from build123d import *

# Parameters (mm, degrees)
STOCK_HORN_DRIVE_FLANGE_START              = 41
STOCK_HORN_DRIVE_FLANGE_PROFILE_R          = 13
STOCK_HORN_DRIVE_FLANGE_PROFILE_R_2        = 4.05
STOCK_HORN_DRIVE_FLANGE_DEPTH              = 3
D_COUPLING_RING_START                      = 44
D_COUPLING_RING_PROFILE_R                  = 7
D_COUPLING_RING_PROFILE_R_2                = 4.05
D_COUPLING_RING_DEPTH                      = 4
D_KEY_LAND_START                           = 44
D_KEY_LAND_PROFILE_W                       = 2.9
D_KEY_LAND_PROFILE_H                       = 4.8
D_KEY_LAND_DEPTH                           = 4
CAPTURED_HORN_KEY_BOSS_START               = 39.35
CAPTURED_HORN_KEY_BOSS_PROFILE_R           = 13
CAPTURED_HORN_KEY_BOSS_DEPTH               = 1.65
KEY_POCKET_HUB_START                       = 39.35
STOCK_HORN_POCKET_HUB_R                    = 3.55
KEY_POCKET_HUB_DEPTH                       = 1.65
KEY_POCKET_HORIZONTAL_START                = 39.35
STOCK_HORN_POCKET_HORIZONTAL_W             = 16.3
STOCK_HORN_POCKET_HORIZONTAL_H             = 4.2
KEY_POCKET_HORIZONTAL_DEPTH                = 1.65
KEY_POCKET_VERTICAL_START                  = 39.35
STOCK_HORN_POCKET_VERTICAL_W               = 4.2
STOCK_HORN_POCKET_VERTICAL_H               = 16.3
KEY_POCKET_VERTICAL_DEPTH                  = 1.65
KEY_POCKET_ROUNDED_TIPS_START              = 39.35
STOCK_HORN_POCKET_ROUNDED_TIPS_R           = 2.1
KEY_POCKET_ROUNDED_TIPS_DEPTH              = 1.65
UNMODIFIED_HORN_CAPTURE_M2_START           = -50
UNMODIFIED_HORN_CAPTURE_M2_PROFILE_R       = 1.15
UNMODIFIED_HORN_CAPTURE_M2_DEPTH           = 102.400389104
HUB_CLEARANCE_IN_KEY_BOSS_ONLY_START       = 39.35
HORN_CENTER_HUB_CLEARANCE_R                = 4
HUB_CLEARANCE_IN_KEY_BOSS_ONLY_DEPTH       = 1.65
YAW_POSITIVE_RETENTION_CROSSBOLT_START     = -10
YAW_POSITIVE_RETENTION_CROSSBOLT_PROFILE_R = 1.1
YAW_POSITIVE_RETENTION_CROSSBOLT_DEPTH     = 62.400389104
CROSSBOLT_FLAT_SEAT_CUT_12_START           = -12
CROSSBOLT_FLAT_SEAT_12_R                   = 2.75
CROSSBOLT_FLAT_SEAT_CUT_12_DEPTH           = 6
CROSSBOLT_FLAT_SEAT_CUT_6_START            = 6
CROSSBOLT_FLAT_SEAT_6_R                    = 2.75
CROSSBOLT_FLAT_SEAT_CUT_6_DEPTH            = 6


with BuildPart() as part:
    # Stock_horn_drive_flange_profile → Stock_horn_drive_flange (new body)
    with BuildSketch(Plane(origin=(0, 0, 0), x_dir=(1, 0, 0), z_dir=(0, 1, 0)).offset(STOCK_HORN_DRIVE_FLANGE_START)):
        with Locations(Location((0, 0, 0), (0, 0, 270))):
            Circle(STOCK_HORN_DRIVE_FLANGE_PROFILE_R)
        with Locations(Location((0, 0, 0), (0, 0, 270))):
            Circle(STOCK_HORN_DRIVE_FLANGE_PROFILE_R_2, mode=Mode.SUBTRACT)
    extrude(amount=STOCK_HORN_DRIVE_FLANGE_DEPTH)

    # D_coupling_ring_profile → D_coupling_ring (add)
    with BuildSketch(Plane(origin=(0, 0, 0), x_dir=(1, 0, 0), z_dir=(0, 1, 0)).offset(D_COUPLING_RING_START)):
        with Locations(Location((0, 0, 0), (0, 0, 270))):
            Circle(D_COUPLING_RING_PROFILE_R)
        with Locations(Location((0, 0, 0), (0, 0, 270))):
            Circle(D_COUPLING_RING_PROFILE_R_2, mode=Mode.SUBTRACT)
    extrude(amount=D_COUPLING_RING_DEPTH)

    # D_key_land_profile → D_key_land (add)
    with BuildSketch(Plane(origin=(0, 0, 0), x_dir=(1, 0, 0), z_dir=(0, 1, 0)).offset(D_KEY_LAND_START)):
        with Locations((4.55, 0)):
            Rectangle(D_KEY_LAND_PROFILE_W, D_KEY_LAND_PROFILE_H)
    extrude(amount=D_KEY_LAND_DEPTH)

    # Captured_horn_key_boss_profile → Captured_horn_key_boss (add)
    with BuildSketch(Plane(origin=(0, 0, 0), x_dir=(1, 0, 0), z_dir=(0, 1, 0)).offset(CAPTURED_HORN_KEY_BOSS_START)):
        with Locations(Location((0, 0, 0), (0, 0, 270))):
            Circle(CAPTURED_HORN_KEY_BOSS_PROFILE_R)
    extrude(amount=CAPTURED_HORN_KEY_BOSS_DEPTH)

    # Stock_horn_pocket_Hub → Key_pocket_Hub (cut)
    with BuildSketch(Plane(origin=(0, 0, 0), x_dir=(1, 0, 0), z_dir=(0, 1, 0)).offset(KEY_POCKET_HUB_START)):
        with Locations(Location((0, 0, 0), (0, 0, 270))):
            Circle(STOCK_HORN_POCKET_HUB_R)
    extrude(amount=KEY_POCKET_HUB_DEPTH, mode=Mode.SUBTRACT)

    # Stock_horn_pocket_Horizontal → Key_pocket_Horizontal (cut)
    with BuildSketch(Plane(origin=(0, 0, 0), x_dir=(1, 0, 0), z_dir=(0, 1, 0)).offset(KEY_POCKET_HORIZONTAL_START)):
        Rectangle(STOCK_HORN_POCKET_HORIZONTAL_W, STOCK_HORN_POCKET_HORIZONTAL_H)
    extrude(amount=KEY_POCKET_HORIZONTAL_DEPTH, mode=Mode.SUBTRACT)

    # Stock_horn_pocket_Vertical → Key_pocket_Vertical (cut)
    with BuildSketch(Plane(origin=(0, 0, 0), x_dir=(1, 0, 0), z_dir=(0, 1, 0)).offset(KEY_POCKET_VERTICAL_START)):
        Rectangle(STOCK_HORN_POCKET_VERTICAL_W, STOCK_HORN_POCKET_VERTICAL_H)
    extrude(amount=KEY_POCKET_VERTICAL_DEPTH, mode=Mode.SUBTRACT)

    # Stock_horn_pocket_Rounded_tips → Key_pocket_Rounded_tips (cut)
    with BuildSketch(Plane(origin=(0, 0, 0), x_dir=(1, 0, 0), z_dir=(0, 1, 0)).offset(KEY_POCKET_ROUNDED_TIPS_START)):
        with Locations((8.15, 0)):
            Circle(STOCK_HORN_POCKET_ROUNDED_TIPS_R)
        with Locations((-8.15, 0)):
            Circle(STOCK_HORN_POCKET_ROUNDED_TIPS_R)
        with Locations((0, 8.15)):
            Circle(STOCK_HORN_POCKET_ROUNDED_TIPS_R)
        with Locations((0, -8.15)):
            Circle(STOCK_HORN_POCKET_ROUNDED_TIPS_R)
    extrude(amount=KEY_POCKET_ROUNDED_TIPS_DEPTH, mode=Mode.SUBTRACT)

    # Unmodified_horn_capture_M2_profile → Unmodified_horn_capture_M2 (cut, through all)
    with BuildSketch(Plane(origin=(0, 0, 0), x_dir=(1, 0, 0), z_dir=(0, 1, 0)).offset(UNMODIFIED_HORN_CAPTURE_M2_START)):
        with Locations(Location((7, 7, 0), (0, 0, 270))):
            Circle(UNMODIFIED_HORN_CAPTURE_M2_PROFILE_R)
        with Locations(Location((-7, 7, 0), (0, 0, 270))):
            Circle(UNMODIFIED_HORN_CAPTURE_M2_PROFILE_R)
        with Locations(Location((-7, -7, 0), (0, 0, 270))):
            Circle(UNMODIFIED_HORN_CAPTURE_M2_PROFILE_R)
        with Locations(Location((7, -7, 0), (0, 0, 270))):
            Circle(UNMODIFIED_HORN_CAPTURE_M2_PROFILE_R)
    extrude(amount=UNMODIFIED_HORN_CAPTURE_M2_DEPTH, mode=Mode.SUBTRACT)

    # Horn_center_hub_clearance → Hub_clearance_in_key_boss_only (cut)
    with BuildSketch(Plane(origin=(0, 0, 0), x_dir=(1, 0, 0), z_dir=(0, 1, 0)).offset(HUB_CLEARANCE_IN_KEY_BOSS_ONLY_START)):
        Circle(HORN_CENTER_HUB_CLEARANCE_R)
    extrude(amount=HUB_CLEARANCE_IN_KEY_BOSS_ONLY_DEPTH, mode=Mode.SUBTRACT)

    # Yaw_positive_retention_crossbolt_profile → Yaw_positive_retention_crossbolt (cut, through all)
    with BuildSketch(Plane(origin=(0, 0, 0), x_dir=(0, 0, -1), z_dir=(1, 0, 0)).offset(YAW_POSITIVE_RETENTION_CROSSBOLT_START)):
        with Locations(Location((0, 45.5, 0), (0, 0, 180))):
            Circle(YAW_POSITIVE_RETENTION_CROSSBOLT_PROFILE_R)
    extrude(amount=YAW_POSITIVE_RETENTION_CROSSBOLT_DEPTH, mode=Mode.SUBTRACT)

    # Crossbolt_flat_seat_-12 → Crossbolt_flat_seat_cut_-12 (cut)
    with BuildSketch(Plane(origin=(0, 0, 0), x_dir=(0, 0, -1), z_dir=(1, 0, 0)).offset(CROSSBOLT_FLAT_SEAT_CUT_12_START)):
        with Locations((0, 45.5)):
            Circle(CROSSBOLT_FLAT_SEAT_12_R)
    extrude(amount=CROSSBOLT_FLAT_SEAT_CUT_12_DEPTH, mode=Mode.SUBTRACT)

    # Crossbolt_flat_seat_6 → Crossbolt_flat_seat_cut_6 (cut)
    with BuildSketch(Plane(origin=(0, 0, 0), x_dir=(0, 0, -1), z_dir=(1, 0, 0)).offset(CROSSBOLT_FLAT_SEAT_CUT_6_START)):
        with Locations((0, 45.5)):
            Circle(CROSSBOLT_FLAT_SEAT_6_R)
    extrude(amount=CROSSBOLT_FLAT_SEAT_CUT_6_DEPTH, mode=Mode.SUBTRACT)


solid = part.part
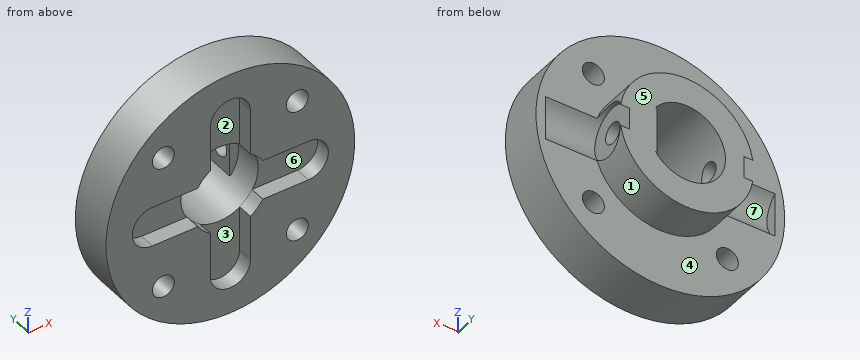
The listing builds one solid part. Answer for the finished solid, in the listing's coordinates (mm). Face numbers are marked on the shaded views. A direction names the side the tool comes from. Coordinates: 2 decimals unless noted, no trailing zeros. Write each loop counter-clockwise with the first axis right and the second up, starting at its lowest first coordinate (ties: lowest second). Pieces come first, ordered by that corner, then holes. Notation, with made-up numbers: (-18, 46.5) - (-5, 46.5) arc R26 cw to (-5, 71.5) - close; hole circle Ø4 at (41, -33.75). An arc over 180 degrees is marked (long way). Answer as CSV lines item,"result".
1. Find section D-D (z = -5.5). Give the vertices of the cut face in (x, y).
Computed values:
outline,"(-11.78, 39.35) - (-2.1, 39.35) - (-2.1, 41) - (2.1, 41) - (2.1, 39.35) - (11.78, 39.35) - (11.78, 44) - (4.33, 44) - (4.33, 48) - (-4.33, 48) - (-4.33, 44) - (-11.78, 44) - close"
2. Determine the mould class of the marked faces 1, 2, 3 and 4 for opening direction X: +X half, -X half, draft (parallel to the pull), parting line (faces both ways), or undercut.
Computed values:
face 1,"parting line"
face 2,"undercut"
face 3,"undercut"
face 4,"draft"
3. Straight lines are drawn through the part: line 1 (X direction, y = 47.25, z = 0); line 2 (X direction, y = 40.6, z = -7); line 3 (Y direction, x = 4.9, z = 0). For each, find the intervals that lie inside material, in ascending order. Write a range as [from, to].
Computed values:
line 1,"x = [-6, -4.05], [3.1, 6]"
line 2,"x = [-10.95, -8.15], [-5.85, -2.1], [2.1, 5.85], [8.15, 10.95]"
line 3,"y = [41, 44.4], [46.6, 48]"
4. Given P1, Ø0.5, axis at y = 40.5, z = -5, coming from the -X side; P2, Ø1.3, axis at y = 45.5, z = 0, coming from the -X side; P3, Ø2, axis at x = -0.5, z = 8, coming from the -Y side; P4, Ø1, axis at x = -4, y = 41, coming from the -Z side, each flat-ended and moving along its own axis, determine where each tip first touches the part or whether it passes through.
Computed values:
P1,"stops at x = -12.1"
P2,"passes through"
P3,"stops at y = 41"
P4,"stops at z = -12.52"
5. Find section C-C (y = 45.5). Give the vertices of the cut face in (x, z).
Computed values:
outline,"(-6.44, -2.75) arc R7 ccw to (6.44, -2.75) - (6, -2.75) - (6, -1.1) - (3.1, -1.1) - (3.1, -2.4) - (3.26, -2.4) arc R4.05 cw to (-3.9, -1.1) - (-6, -1.1) - (-6, -2.75) - close; (-6.44, 2.75) - (-6, 2.75) - (-6, 1.1) - (-3.9, 1.1) arc R4.05 cw to (3.26, 2.4) - (3.1, 2.4) - (3.1, 1.1) - (6, 1.1) - (6, 2.75) - (6.44, 2.75) arc R7 ccw to start"
6. A tool of negligible diameter and unlimited length cuts with its end or side. For the marked faces 5, 6 and 7, from which of +Z, -Z, +X, -X, +Y, -Y can it reach the whole face along a straight path? Write none if from no direction.
Computed values:
face 5,"+Z, -Z, +X, -X, +Y"
face 6,"-Y"
face 7,"none"
7. Find section A-A (x = 0). Give the vertices of the cut face in (y, z).
Computed values:
outline,"(39.35, -13) - (44, -13) - (44, -7) - (48, -7) - (48, -4.05) - (41, -4.05) - (41, -10.25) - (39.35, -10.25) - close; (39.35, 10.25) - (41, 10.25) - (41, 4.05) - (48, 4.05) - (48, 7) - (44, 7) - (44, 13) - (39.35, 13) - close"
8. Find section B-B (y = 40.25). Give the vertices of the cut face in (x, z), plus the area to 3 significant figures.
Computed values:
outline,"circle Ø26 at (0, 0); hole circle Ø2.3 at (-7, -7); hole (-8.15, -2.1) - (-3.4, -2.1) arc R4 ccw to (-2.1, -3.4) - (-2.1, -8.15) arc R2.1 ccw to (2.1, -8.15) - (2.1, -3.4) arc R4 ccw to (3.4, -2.1) - (8.15, -2.1) arc R2.1 ccw to (8.15, 2.1) - (3.4, 2.1) arc R4 ccw to (2.1, 3.4) - (2.1, 8.15) arc R2.1 ccw to (-2.1, 8.15) - (-2.1, 3.4) arc R4 ccw to (-3.4, 2.1) - (-8.15, 2.1) arc R2.1 ccw to start; hole circle Ø2.3 at (-7, 7); hole circle Ø2.3 at (7, -7); hole circle Ø2.3 at (7, 7)"
area,"363 mm²"
